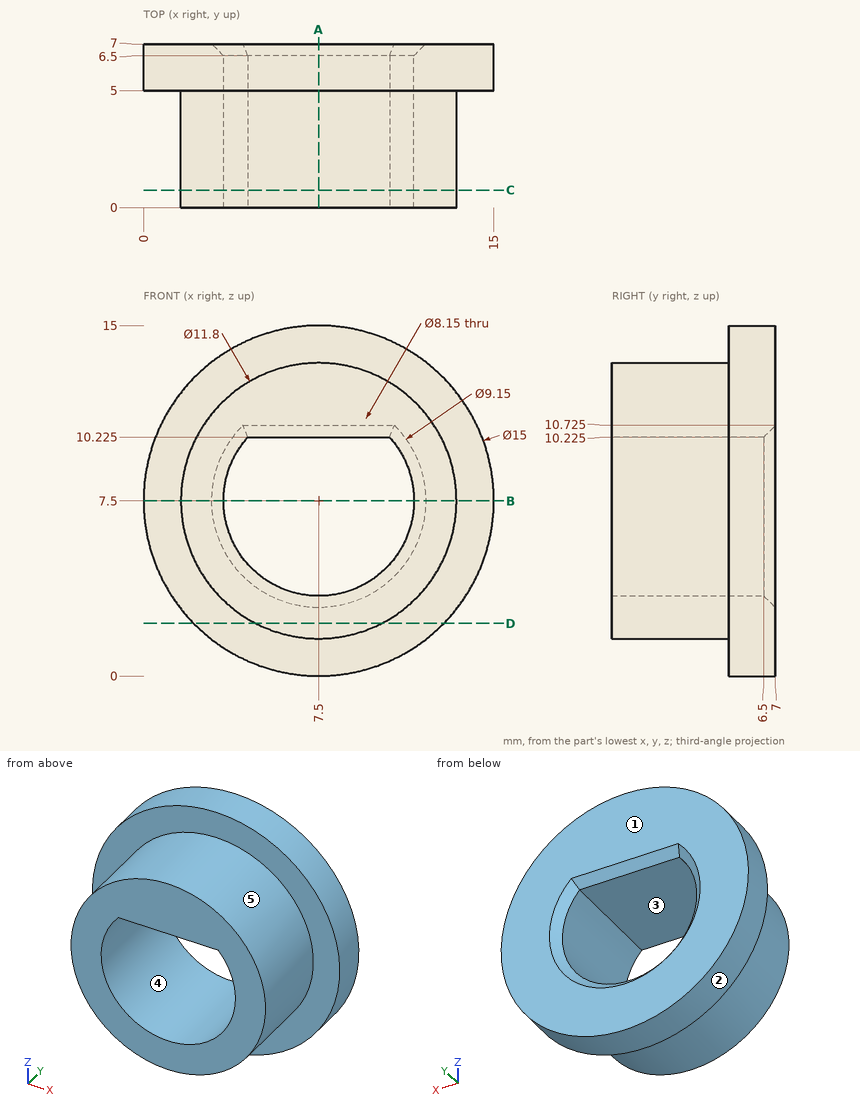
Input: dimensioned drawing with shaded views. Units: mm. Origin: part minimum x, y, z. A direction names the side the tool comes from. Give positions to 0.01 mm unless a question says otherwise; leave off trailing zeros. Loops run counter-clockwise (first coordinate to the right, second up) from the corner with the lowest first, then second, coordinate; pieces in that order, holes last. Notation, with made-up numbers: (-2, 12.5) -> (10, 12.5) arc R16 ccw to (10, 33.5) -> close; hole circle Ø5 at (83.25, 42.5). An arc over 180 degrees is marked (long way). Use a Markdown table: item, result. Add a question column.
1) Pull-direction query (X, two-part tool) for the marked faces 1, 2 and 3; classes: +X half, -X half, draft (parallel to the pull), parting line (faces both ways), or undercut.
2) First-contact query: pin 1 (1 mm diameter, centred on y = 3, z = 7.5, fed in from -X); pin 2 (1.8 mm diameter, centred on x = 8, y = 3.5, fed in from -Z); pin 3 (1 mm diameter, centred on x = 12.5, y = 1, fed in from +Z). Flat tips, straight axial feed; report the tip coordinate or a pass-through.
3) Section query A-A, the plane x = 7.5. Return the cut outline in (y, z) (3 decimals), then the cut area to 4 significant figures.
4) Reachability of the marked faces 4 and 5 from +Z, -Z, +X, -X, +Y, -Y: full face, straight path, thin tool, end or side. Return the list, or none.
5) Section query C-C, the plane y = 0.75. Return the cut outline in (x, z) (3 decimals).
6) Section query B-B, the plane z = 7.5. Return the cut outline in (x, y) (3 decimals), then the cut area to 3 significant figures.
7) Line query: line 1 along X through (y, z) = (5.25, 7.5) (3 decimals); line 2 along Y through (x, z) = (1.5, 7.5); line 3 along Z through (x, y) = (8.75, 2.5) (3 decimals). Output: solid intervals per line, ascending. Write a range as [from, to].
8) Section query D-D, the plane z = 2.25. Return the cut outline in (x, y), then the cut area to 3 significant figures.
Numbers:
| question | item | result |
|---|---|---|
| 1 | face 1 | draft |
| 1 | face 2 | parting line |
| 1 | face 3 | undercut |
| 2 | pin 1 | stops at x = 1.6 |
| 2 | pin 2 | stops at z = 1.6 |
| 2 | pin 3 | stops at z = 11.32 |
| 3 | outline | (0, 1.6) -> (5, 1.6) -> (5, 0) -> (7, 0) -> (7, 2.925) -> (6.5, 3.425) -> (0, 3.425) -> close; (0, 10.225) -> (6.5, 10.225) -> (7, 10.725) -> (7, 15) -> (5, 15) -> (5, 13.4) -> (0, 13.4) -> close |
| 3 | area | 41.15 mm2 |
| 4 | face 4 | +Y, -Y |
| 4 | face 5 | -Y |
| 5 | outline | circle Ø11.8 at (7.5, 7.5); hole (4.47, 10.225) arc R4.075 ccw (long way) to (10.53, 10.225) -> close |
| 6 | outline | (0, 5) -> (1.6, 5) -> (1.6, 0) -> (3.425, 0) -> (3.425, 6.5) -> (2.925, 7) -> (0, 7) -> close; (11.575, 0) -> (13.4, 0) -> (13.4, 5) -> (15, 5) -> (15, 7) -> (12.075, 7) -> (11.575, 6.5) -> close |
| 6 | area | 31.7 mm2 |
| 7 | line 1 | x = [0, 3.425], [11.575, 15] |
| 7 | line 2 | y = [5, 7] |
| 7 | line 3 | z = [1.734, 3.621], [10.225, 13.266] |
| 8 | outline | (2.14, 5) -> (4.81, 5) -> (4.81, 0) -> (10.19, 0) -> (10.19, 5) -> (12.86, 5) -> (12.86, 7) -> (2.14, 7) -> close |
| 8 | area | 48.3 mm2 |
